Verification items for the finished model (mm, model axes). Face numbers are marked on the shaded views. A direction names the side the tool comes from. Give positions to 0.01 mm unless a question says otherwise; leave off trailing zeros. Order: outer loops, then holes, each group sorted by start corner. A loop starts at its lowest first (then second) coordinate and runs counter-clockwise, first axis right, second up.
(1) Scan lines: L1, parallel to X at y = 4.3, z = 0 (3 decimals); L2, parallel to X at y = 1.25, z = 0.5; L3, parallel to Z at x = 23, y = 4.65 (3 decimals). Record each from-to range of solid material in increasing order.
(2) Sectioned sample at D-D on z = 0.5. Count the separate pieces of the cut face and the enclosed holes in it, plus the area to 3 significant figures.
(3) Sectioned sample at B-B on x = 11. Record the cut outline in (y, z), plus the area to 3 significant figures.
(4) Access from +Z, -Z, +X, -X, +Y, -Y to the whole of each face (thin tool, end or side, straight path). Record for the marked faces 3, 4 and 5.
(5) Sectioned sample at C-C on y = 2.1. Record the cut outline in (x, z).
(6) Mould release check, pull along X, two halves, no side actions. Record for the marked faces 1 and 2: pulls with the +X half, pulls with the -X half, needs draft (parallel to the pull), parting line crosses it, or undercut.
(7) Gauge pin test, flat ends, axial feed: pin 1 (5 mm diameter, centred on x = 0, z = 0, fed in from +Y); pin 2 (2 mm diameter, centred on y = 2, z = 2.5, fed in from -X); pin 3 (2.5 mm diameter, centred on x = 24, z = 1.5, fed in from -Y). Record the tip position at first contact, or that the pin passes through.
(8) Sectioned sample at A-A on y = 5.1. Record the cut outline in (x, z) (3 decimals).
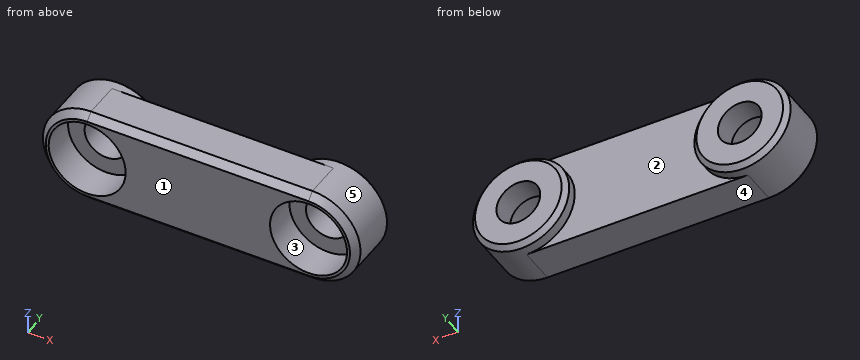
```python
from build123d import *

# Parameters (mm, degrees)
EXTRUDE_1_DEPTH     = 6
CUT_EXTRUDE_START   = -1.5
SKETCH_4_W          = 74.791186833
SKETCH_4_H          = 47.147225829
SKETCH_4_R          = 5
CUT_EXTRUDE_1_DEPTH = 1.5
CHAMFER_1_SIZE      = 0.5
CHAMFER_2_SIZE      = 0.7


with BuildPart() as part:
    # 草图1 → 凸台-拉伸1 (new body)
    with BuildSketch(Plane(origin=(0, 0, 0), x_dir=(1, 0, 0), z_dir=(0, 1, 0))):
        with BuildLine():
            Line((0, 5), (23, 5))
            ThreePointArc((23, 5), (28, 0), (23, -5))
            Line((23, -5), (0, -5))
            ThreePointArc((0, -5), (-5, 0), (0, 5))
        make_face()
    extrude(amount=EXTRUDE_1_DEPTH)

    # 草图2 → 切除-旋转1 (revolve, cut)
    with BuildSketch(Plane.XY, mode=Mode.PRIVATE) as cut_revolve_1_sk:
        Polygon((-4, 0), (-4, 3.5), (-2.275, 3.5), (-2.275, 6), (0, 6), (0, 0), align=None)
    revolve(cut_revolve_1_sk.sketch.rotate(Axis((0, 0, 0), (0, 1, 0)), 270), axis=Axis((0, 0, 0), (0, 1, 0)), mode=Mode.SUBTRACT)

    # 草图3 → 切除-旋转2 (revolve, cut)
    with BuildSketch(Plane.XY, mode=Mode.PRIVATE) as cut_revolve_2_sk:
        Polygon((23, 0), (19, 0), (19, 3.5), (20.725, 3.5), (20.725, 6), (23, 6), align=None)
    revolve(cut_revolve_2_sk.sketch.rotate(Axis((23, 0, 0), (0, 1, 0)), 270), axis=Axis((23, 0, 0), (0, 1, 0)), mode=Mode.SUBTRACT)

    # 草图4 → 切除-拉伸1 (cut)
    with BuildSketch(Plane(origin=(0, 6, 0), x_dir=(1, 0, 0), z_dir=(0, 1, 0)).offset(CUT_EXTRUDE_START)):
        with Locations((14.679246855, 1.415799858)):
            Rectangle(SKETCH_4_W, SKETCH_4_H)
        with Locations(Location((23, 0, 0), (0, 0, 270))):
            Circle(SKETCH_4_R, mode=Mode.SUBTRACT)
        with Locations(Location((0, 0, 0), (0, 0, 270))):
            Circle(SKETCH_4_R, mode=Mode.SUBTRACT)
    extrude(amount=CUT_EXTRUDE_1_DEPTH, mode=Mode.SUBTRACT)

    # 倒角1
    chamfer_1_edges = [part.edges().sort_by_distance(p)[0] for p in [
        (23, 6, 5),
        (0, 6, -5),
    ]]
    chamfer(chamfer_1_edges, length=CHAMFER_1_SIZE)

    # 倒角2
    chamfer_2_edges = [part.edges().sort_by_distance(p)[0] for p in [
        (11.5, 0, -5),
        (28, 0, 0),
        (11.5, 0, 5),
        (-5, 0, 0),
    ]]
    chamfer(chamfer_2_edges, length=CHAMFER_2_SIZE)


solid = part.part
```
Ans:
1. L1: x = -5 to -2.275, 2.275 to 20.725, 25.275 to 28
1. L2: x = -4.97 to -3.97, 3.97 to 19.03, 26.97 to 27.97
1. L3: z = -5 to -2.275, 2.275 to 5
2. separate pieces: 3
2. enclosed holes: 0
2. area: 99.4 mm2
3. outline: (0, -4.3) - (0.7, -5) - (4.5, -5) - (4.5, 5) - (0.7, 5) - (0, 4.3) - close
3. area: 44.5 mm2
4. face 3: -Y
4. face 4: -Z, +X, -X, +Y, -Y
4. face 5: +Y
5. outline: (0, -5) - (23, -5) arc R5 ccw to (23, 5) - (0, 5) arc R5 ccw to start; hole circle Ø8 at (0, 0); hole circle Ø8 at (23, 0)
6. face 1: needs draft
6. face 2: undercut
7. pin 1: stops at y = 6
7. pin 2: stops at x = -4.77
7. pin 3: stops at y = 3.5
8. outline: circle Ø10 at (0, 0); circle Ø10 at (23, 0); hole circle Ø4.55 at (0, 0); hole circle Ø4.55 at (23, 0)
